Can you work these out from the model? Positions are in its coordinate system, mm. Face numbers are marked on the shaded views. A direction names the side the tool comes from. Round coordinates to 2 decimals unless told otherwise and drop trailing zeros. Order: outer loops, then holes, each group sorted by start corner. A loop starts at its lowest first (then second) coordinate and runs counter-clockwise, first axis right, second up.
Q1. If we section it at C-C (x = -10.5): Please give me the cut outline in (y, z).
Q2. If we section it at A-A (y = 0): Please give me the cut outline in (x, z), plus the area to 3 significant figures.
Q3. If I drill on line 1 (X direction, y = -21.5, z = -25); line 2 (Z direction, x = 9, y = 0), over which ranges is the centre line in solid material (lowest first)?
Q4. For the marked faces 1 and 2, which set-ups out of +Z, -Z, +X, -X, +Y, -Y let a thin tool reach every point of the face, with its end or its side?
Q5. We'd pull the mould along X, two halves only. Please class the marked faces 3, 4 and 5: pulls with the +X half, pulls with the -X half, needs draft (parallel to the pull), parting line crosses it, or undercut.
Q6. If we section it at D-D (z = 17): Please give me the cut outline in (x, y).
Q7. Will these pins go through, and if not, where does the flat tip stop? P1, Ø2, axis at x = -2.5, y = -14, coming from the +Z side; P2, Ø5, axis at x = 5, z = -2.5, coming from the -Y side; P3, Ø3, axis at x = 15, y = 20, coming from the +Z side.
from build123d import *

# Parameters (mm, degrees)
F0_R     = 25
F1_DEPTH = 20
F2_R     = 37.5
F2_R_2   = 25
F3_DEPTH = 5
F6_D     = 20
F6_DEPTH = 250


with BuildPart() as f1:
    # F0 (on Right) → F1 (new body)
    with BuildSketch(Plane.YZ):
        Circle(F0_R)
    extrude(amount=F1_DEPTH)

    # F2 (on face) → F3 (join)
    with BuildSketch(Plane.YZ.offset(20)):
        Circle(F2_R)
        Circle(F2_R_2, mode=Mode.SUBTRACT)
        Circle(F2_R_2)
    extrude(amount=F3_DEPTH)

    # F4: F1 across face


with BuildPart() as f1_1:
    add(f1.part)
    add(f1.part.mirror(Plane(origin=(0, 0, 0), x_dir=(0, 1, 0), z_dir=(-1, 0, 0))))

    # F6
    with Locations(Plane.YZ.offset(25)):
        with Locations((0, 0)):
            Hole(F6_D / 2, depth=F6_DEPTH)


solid = f1_1.part
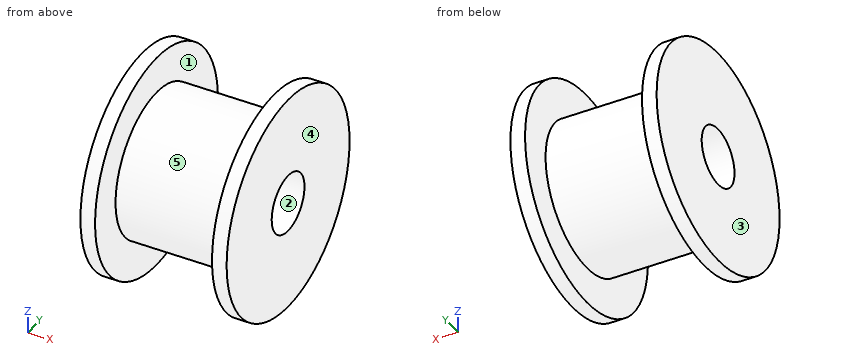
Solution:
1. outline: circle Ø50 at (0, 0); hole circle Ø20 at (0, 0)
2. outline: (-25, -37.5) - (-20, -37.5) - (-20, -25) - (20, -25) - (20, -37.5) - (25, -37.5) - (25, -10) - (-25, -10) - close; (-25, 10) - (25, 10) - (25, 37.5) - (20, 37.5) - (20, 25) - (-20, 25) - (-20, 37.5) - (-25, 37.5) - close
2. area: 1,750 mm2
3. line 1: x = -25 to -20, 20 to 25
3. line 2: z = -25 to -10, 10 to 25
4. face 1: none
4. face 2: +X, -X
5. face 3: pulls with the -X half
5. face 4: pulls with the +X half
5. face 5: undercut
6. outline: (-25, -33.43) - (-20, -33.43) - (-20, -18.33) - (20, -18.33) - (20, -33.43) - (25, -33.43) - (25, 33.43) - (20, 33.43) - (20, 18.33) - (-20, 18.33) - (-20, 33.43) - (-25, 33.43) - close
7. P1: stops at z = 21.35
7. P2: stops at y = -25
7. P3: stops at z = 16.82
